Model file for the job. Use its own axes, mm. Round coordinates to 2 decimals unless told otherwise and drop trailing zeros. Loops run counter-clockwise (first coordinate to the right, second up) from the corner with the lowest first, then second, coordinate; pieces in that order, holes last.
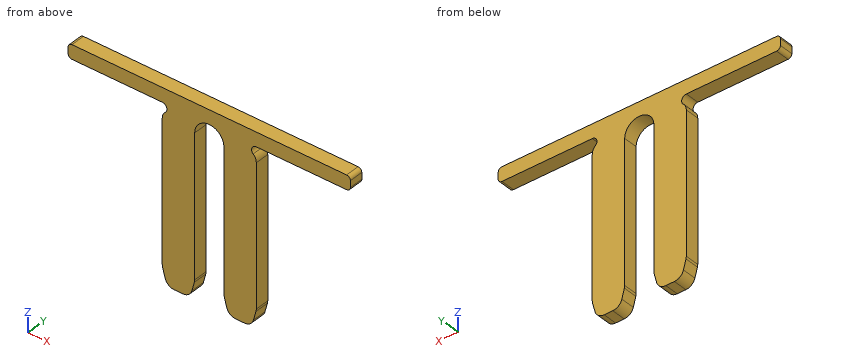
from build123d import *

# Parameters (mm, degrees)
PAD013_DEPTH = 0.75
FILLET018_R  = 0.4
FILLET019_R  = 1


with BuildPart() as part:
    # Sketch016 → Pad013 (new body, symmetric)
    with BuildSketch(Plane.XZ):
        with BuildLine():
            Line((-15, 10), (15, 10))
            Line((15, 10), (15, 8.5))
            Line((15, 8.5), (6, 8.5))
            Line((6, 8.5), (5, 8.5))
            ThreePointArc((5, 8.5), (4.5, 8), (5, 7.5))
            Line((5, 7.5), (5, -8.133975))
            Line((5, -8.133975), (4.5, -10))
            Line((2.05, -10), (4.5, -10))
            Line((1.55, -8.133975), (2.05, -10))
            Line((1.55, 6.95), (1.55, -8.133975))
            ThreePointArc((1.55, 6.95), (0, 8.5), (-1.55, 6.95))
            Line((-1.55, -8.133975), (-1.55, 6.95))
            Line((-1.55, -8.133975), (-2.05, -10))
            Line((-4.5, -10), (-2.05, -10))
            Line((-5, -8.133975), (-4.5, -10))
            Line((-5, 7.5), (-5, -8.133975))
            ThreePointArc((-5, 7.5), (-4.5, 8), (-5, 8.5))
            Line((-6, 8.5), (-5, 8.5))
            Line((-15, 8.5), (-6, 8.5))
            Line((-15, 8.5), (-15, 10))
        make_face()
    extrude(amount=PAD013_DEPTH, both=True)

    # Fillet018
    fillet018_edges = [part.edges().sort_by_distance(p)[0] for p in [
        (-15, 0, 10),
        (-15, 0, 8.5),
        (15, 0, 10),
        (15, 0, 8.5),
    ]]
    fillet(fillet018_edges, radius=FILLET018_R)

    # Fillet019
    fillet019_edges = [part.edges().sort_by_distance(p)[0] for p in [
        (-5, 0, 7.5),
        (-5, 0, -8.133975),
        (-4.5, 0, -10),
        (-2.05, 0, -10),
        (-1.55, 0, -8.133975),
        (1.55, 0, -8.133975),
        (2.05, 0, -10),
        (4.5, 0, -10),
        (5, 0, -8.133975),
        (5, 0, 7.5),
    ]]
    fillet(fillet019_edges, radius=FILLET019_R)


solid = part.part
Q1. Flat gauge pin, fed straight in: P1, Ø0.8, axis at y = 0.5, z = -1, coming from the -X side. Where does the tip first touch, or does it go through?
Q2. Slice it at C-C on z = 7.25. Give the cut face in (x, y), plus the area to 3 significant figures.
Q3. Probe line 1 (X direction, y = -0.05, z = -7.25); line 2 (Z direction, x = 7.5, y = -0.3). List the from-to ranges inside material, lowest first.
Q4. Slice it at D-D on x = -12. Give the cut face in (y, z).
Q5. Slice it at A-A on z = -7. Give the cut face in (x, y), plus the area to 4 significant figures.
Reply:
1. P1: stops at x = -5
2. outline: (-4.93, -0.75) - (-1.52, -0.75) - (-1.52, 0.75) - (-4.93, 0.75) - close; (1.52, -0.75) - (4.93, -0.75) - (4.93, 0.75) - (1.52, 0.75) - close
2. area: 10.2 mm2
3. line 1: x = -5 to -1.55, 1.55 to 5
3. line 2: z = 8.5 to 10
4. outline: (-0.75, 8.5) - (0.75, 8.5) - (0.75, 10) - (-0.75, 10) - close
5. outline: (-5, -0.75) - (-1.55, -0.75) - (-1.55, 0.75) - (-5, 0.75) - close; (1.55, -0.75) - (5, -0.75) - (5, 0.75) - (1.55, 0.75) - close
5. area: 10.35 mm2
